Verification items for the finished model (mm, model axes). A direction names the side the tool comes from. Round coordinates to 2 decimals unless told otherwise and drop trailing zeros. Order: outer loops, then holes, each group sorted by start corner. A loop starts at its lowest first (then second) coordinate and runs counter-clockwise, first axis right, second up. Notation, with made-up numbers: (-35, 11) -> (-10, 11) arc R18 cw to (-10, 25) -> close; hole circle Ø4 at (5, 85). An arc over 180 degrees is marked (long way). Put each result on its own line as item: value.
Autodesk Inventor part; units mm, degrees
ref_plane "YZ Plane" through (0, 0, 0) normal (1, 0, 0) x (0, 1, 0)
ref_plane "XZ Plane" through (0, 0, 0) normal (0, 1, 0) x (-1, 0, 0)
ref_plane "XY Plane" through (0, 0, 0) normal (0, 0, 1) x (1, 0, 0)
sketch "Sketch1" plane through (0, 0, 0) normal (0, 0, 1) x (1, 0, 0)
  circle A0 centre (-2, 20.4853) radius 4.25
  circle A1 centre (124.1, 20.4853) radius 4.25
  line L0 (-17, 26.4853) -> (-17, 14.4853)
  line L1 (-17, 26.4853) -> (-8.5147, 34.9706)
  line L2 (-17, 14.4853) -> (-8.5147, 6)
  line L3 (-8.5147, 34.9706) -> (130.6147, 34.9706)
  line L4 (130.6147, 34.9706) -> (139.1, 26.4853)
  line L5 (139.1, 26.4853) -> (139.1, 14.4853)
  line L6 (139.1, 14.4853) -> (130.6147, 6)
  circle A2 centre (-2, 20.4853) radius 13 construction
  circle A3 centre (-2, 20.4853) radius 17 construction
  line L7 (-8.5147, 6) -> (0, 6)
  line L8 (0, 6) -> (0, 0)
  line L9 (130.6147, 6) -> (122.1, 6)
  line L10 (122.1, 6) -> (122.1, 0)
  line L11 (122.1, 0) -> (0, 0)
  point P0 (0, 0)
  point P1 (-17, 20.4853)
  dimension "d0" = 8.5
  dimension "d1" = 126.1
  dimension "d2" = 45
  dimension "d3" = 12
  dimension "d4" = 26
  dimension "d5" = 34
  dimension "d6" = 15
  dimension "d7" = 6
  dimension "d10" = 15
  dimension "d18" = 2
extrude "Extrusion1" add sketch "Sketch1" along normal blind 6
sketch "Sketch2" plane through (0, 0, 6) normal (0, 0, 1) x (1, 0, 0)
  line L0 (130.6147, 34.9706) -> (-8.5147, 34.9706)
  line L1 (-8.5147, 34.9706) -> (-17, 26.4853)
  line L2 (3.4853, 34.9706) -> (11.9706, 26.4853)
  line L3 (11.9706, 26.4853) -> (110.1294, 26.4853)
  line L4 (110.1294, 26.4853) -> (118.6147, 34.9706)
  point P0 (-17, 14.4853)
  dimension "d13" = 12
  dimension "d14" = 12
  dimension "d15" = 12
extrude "Extrusion2" cut sketch "Sketch2" against normal blind 6
sketch "Sketch3" plane through (0, 0, 6) normal (0, 0, 1) x (1, 0, 0)
  line L0 (0, 0) -> (122.1, 0)
  line L1 (110.1294, 26.4853) -> (11.9706, 26.4853)
  line L2 (57.05, 16) -> (65.05, 16)
  line L3 (65.05, 16) -> (65.05, 10)
  line L4 (65.05, 10) -> (57.05, 10)
  line L5 (57.05, 10) -> (57.05, 16)
  line L6 (27.05, 16) -> (35.05, 16)
  line L7 (35.05, 16) -> (35.05, 10)
  line L8 (35.05, 10) -> (27.05, 10)
  line L9 (27.05, 10) -> (27.05, 16)
  line L10 (87.05, 16) -> (95.05, 16)
  line L11 (95.05, 16) -> (95.05, 10)
  line L12 (95.05, 10) -> (87.05, 10)
  line L13 (87.05, 10) -> (87.05, 16)
  point P0 (61.05, 16)
  point P1 (61.05, 26.4853)
  dimension "d20" = 8
  dimension "d21" = 6
  dimension "d22" = 8
  dimension "d23" = 8
  dimension "d24" = 10
  dimension "d25" = 22
  dimension "d26" = 22
extrude "Extrusion3" cut sketch "Sketch3" against normal through all
sketch "Sketch4" plane through (0, 0, 6) normal (0, 0, 1) x (1, 0, 0)
  line L0 (0, 0) -> (122.1, 0)
  line L1 (13.1, 0) -> (21.1, 0)
  line L2 (21.1, 0) -> (21.1, -4)
  line L3 (19.1, -6) -> (15.1, -6)
  line L4 (13.1, -4) -> (13.1, 0)
  line L5 (51.1, 0) -> (59.1, 0)
  line L6 (59.1, 0) -> (59.1, -4)
  line L7 (57.1, -6) -> (53.1, -6)
  line L8 (51.1, -4) -> (51.1, 0)
  line L9 (89.1, 0) -> (97.1, 0)
  line L10 (97.1, 0) -> (97.1, -4)
  line L11 (95.1, -6) -> (91.1, -6)
  line L12 (89.1, -4) -> (89.1, 0)
  arc A0 (13.1, -4) -> (15.1, -6) centre (15.1, -4) ccw
  arc A1 (19.1, -6) -> (21.1, -4) centre (19.1, -4) ccw
  arc A2 (51.1, -4) -> (53.1, -6) centre (53.1, -4) ccw
  arc A3 (57.1, -6) -> (59.1, -4) centre (57.1, -4) ccw
  arc A4 (89.1, -4) -> (91.1, -6) centre (91.1, -4) ccw
  arc A5 (95.1, -6) -> (97.1, -4) centre (95.1, -4) ccw
  dimension "d29" = 2
  dimension "d30" = 8
  dimension "d31" = 8
  dimension "d32" = 8
  dimension "d33" = 6
  dimension "d34" = 6
  dimension "d35" = 6
  dimension "d36" = 25
  dimension "d37" = 30
  dimension "d38" = 30
extrude "Extrusion4" add sketch "Sketch4" against normal blind 6
chamfer "Chamfer1" distance 2 angle 45 2 edges at (0, 6, 3) (122.1, 6, 3)
equation "\"d14\" = d13"
equation "\"d15\" = d14"
equation "\"d26\" = d25"
properties part number "rope_mount_b"
Item 1: Section check A-A on x = 30. Record the boundary of the cut face in (y, z), then the cut area to 3 significant figures.
Check sheet entries:
outline: (0, 0) -> (10, 0) -> (10, 6) -> (0, 6) -> close; (16, 0) -> (26.49, 0) -> (26.49, 6) -> (16, 6) -> close
area: 123 mm^2
Item 2: Section check B-B on z = 4.3. State how many separate pieces and enclosed holes the cut face has, then the cut area to 3 significant figures.
Check sheet entries:
separate pieces: 1
enclosed holes: 5
area: 4,090 mm^2
Item 3: Material ranges on L1, parallel to X at y = -3, z = 5.6; L2, parallel to X at y = 23, z = 1.2; L3, parallel to Y at x = -2, z = 3.6, recorded low to high. Write a range as [from, to].
Check sheet entries:
L1: x = [13.1, 21.1], [51.1, 59.1], [89.1, 97.1]
L2: x = [-17, -5.43], [1.43, 120.67], [127.53, 139.1]
L3: y = [6, 16.24], [24.74, 34.97]
Item 4: Tool access check on faces 1 (the flat face through (74, 0, 3)), 2 (the flat face through (65.05, 13, 3)), 3 (the flat face through (0, 2, 3)), 4 (the flat face through (60, 26.485, 3)). Record the directions out of +Z, -Z, +X, -X, +Y, -Y that give a thin tool (end or side, any length) a straight path to the whole face; none if there is none.
Check sheet entries:
face 1: +Z, -Z, -Y
face 2: +Z, -Z
face 3: +Z, -Z, -X, -Y
face 4: +Z, -Z, +Y
Item 5: Gauge pin test, flat ends, axial feed: pin 1 Ø1.2 at (y, z) = (-2.5, 4) entering from -X; pin 2 Ø1.8 at (x, z) = (59.5, 3.5) entering from +Y; pin 3 Ø1 at (y, z) = (13, 1) entering from +X. Record the tip position at first contact, or that the pin passes through.
Check sheet entries:
pin 1: stops at x = 13.1
pin 2: stops at y = 26.49
pin 3: stops at x = 138.11
